```python
from build123d import *

# Parameters (mm, degrees)
RESSALTO_EXTRUS_O1_DEPTH     = 58
ESBO_O3_R                    = 2.75
RESSALTO_EXTRUS_O2_DEPTH     = 9
FILETE1_R                    = 5
FURO_DE_DI_METRO_0_15_14_1_D = 14
FUROAVAN_ADO1_OUTLINE_R      = 4.75
FUROAVAN_ADO1_DEPTH          = 9


# Read off the part's stored shape, not the designer's step: FuroAvançado1
with BuildPart() as part:
    # Esboço2 → Ressalto-extrusão1 (new body)
    with BuildSketch(Plane.XY):
        Polygon((-58, 0), (0, 0), (58, 0), (58, 9), (0, 9), (-58, 9), align=None)
    extrude(amount=-RESSALTO_EXTRUS_O1_DEPTH)

    # Esboço3 → Ressalto-extrusão2 (add)
    with BuildSketch(Plane(origin=(0, 9, 0), x_dir=(1, 0, 0), z_dir=(0, 1, 0))):
        with BuildLine():
            Line((-43.5, 42), (-24.799193535, 42))
            ThreePointArc((-24.799193535, 42), (0, 57), (24.799193535, 42))
            Line((24.799193535, 42), (43.5, 42))
            ThreePointArc((43.5, 42), (56.5, 29), (43.5, 16))
            Line((43.5, 16), (24.799193535, 16))
            ThreePointArc((24.799193535, 16), (0, 1), (-24.799193535, 16))
            Line((-24.799193535, 16), (-43.5, 16))
            ThreePointArc((-43.5, 16), (-56.5, 29), (-43.5, 42))
        make_face()
        with Locations(Location((-11, 42, 0), (0, 0, 270))):
            Circle(ESBO_O3_R, mode=Mode.SUBTRACT)
        with Locations(Location((11, 42, 0), (0, 0, 270))):
            Circle(ESBO_O3_R, mode=Mode.SUBTRACT)
        with Locations(Location((-11, 16, 0), (0, 0, 270))):
            Circle(ESBO_O3_R, mode=Mode.SUBTRACT)
        with Locations(Location((11, 16, 0), (0, 0, 270))):
            Circle(ESBO_O3_R, mode=Mode.SUBTRACT)
    extrude(amount=RESSALTO_EXTRUS_O2_DEPTH)

    # Filete1
    filete1_edges = [part.edges().sort_by_distance(p)[0] for p in [
        (24.799193535, 13.5, -42),
        (-24.799193535, 13.5, -42),
        (-24.799193535, 13.5, -16),
        (24.799193535, 13.5, -16),
    ]]
    fillet(filete1_edges, radius=FILETE1_R)

    # Furo de diâmetro Ø0.15 (14)1 (through all)
    with Locations(Plane(origin=(0, 18, 0), x_dir=(1, 0, 0), z_dir=(0, 1, 0))):
        with Locations((-43.5, 29), (43.5, 29)):
            Hole(FURO_DE_DI_METRO_0_15_14_1_D / 2)

    # FuroAvançado1 outline → FuroAvançado1 (cut)
    with BuildSketch(Plane(origin=(0, 0, 0), x_dir=(1, 0, 0), z_dir=(0, 1, 0))):
        with Locations((-11, 42)):
            Circle(FUROAVAN_ADO1_OUTLINE_R)
        with Locations((-11, 16)):
            Circle(FUROAVAN_ADO1_OUTLINE_R)
        with Locations((11, 16)):
            Circle(FUROAVAN_ADO1_OUTLINE_R)
        with Locations((11, 42)):
            Circle(FUROAVAN_ADO1_OUTLINE_R)
    extrude(amount=FUROAVAN_ADO1_DEPTH, mode=Mode.SUBTRACT)


solid = part.part
```
Model file for the job. Use its own axes, mm. A direction names the side the tool comes from. Coordinates: 2 decimals unless noted, no trailing zeros. Order: outer loops, then holes, each group sorted by start corner. A loop starts at its lowest first (then second) coordinate and runs counter-clockwise, first axis right, second up. Notation, with made-up numbers: (22, -37.75) - (81, -37.75) arc R19 cw to (81, -4.75) - close; hole circle Ø2 at (20, 79.25). An arc over 180 degrees is marked (long way). Return JSON: item names as keys, results as strings. Group by question number.
1) Probe line 1 (Z direction, x = -11, y = 7); line 2 (X direction, y = 6.25, z = -16); line 3 (X direction, y = 10.5, z = -18.5). List the from-to ranges inside material, lowest first. Write a range as from..to.
2) Saw through at A-A, the plane y = 15.5. Write the cut outline in (x, z).
3) Tool access for faces 1 (the flat face through (-8, 9, -16)), 2 (the flat face through (35, 13, -42)), 3 (the flat face through (-36, 13, -42)): list every direction of +Z, -Z, +X, -X, +Y, -Y with a clear straight run to the whole face (end or side of a thin tool).
4) Saw through at D-D, the plane z = -10. Write the cut outline in (x, y), plus the area to 3 significant figures.
5) Saw through at C-C, the plane z = -24.5. Write the cut outline in (x, y), plus the area to 3 significant figures.
6) Flat gauge pins, fed straight in: P1, Ø3, axis at x = -4.5, y = 11.5, coming from the +Z side; P2, Ø5, axis at x = 12, z = -17, coming from the -Y side; P3, Ø4.5, axis at x = -11, z = -42, coming from the +Y side; P4, Ø2.5, axis at x = -37, y = 14, coming from the -Z side. Where does each tip first touch, or does it go through?
7) Saw through at B-B, the plane x = 11. Write the cut outline in (y, z).
8) Mould opens along Z. For faces 4 (the cylindrical face through (10.38, 4.44, -20.71)), 5 (the cylindrical face through (25.244, 13.563, -15.379)), 6 (the cylindrical face through (-56.497, 13.437, -28.714)) say: released by +Z, released by -Z, zero draft, split by the parting line, or undercut.
Values found:
{
 "1": {"line 1": "z = -58..-46.75, -37.25..-20.75, -11.25..0", "line 2": "x = -58..-15.75, -6.25..6.25, 15.75..58", "line 3": "x = -51.16..-12.15, -9.85..9.85, 12.15..51.16"},
 "2": {"outline": "(-43.5, -42) - (-27.66, -42) arc R5 cw to (-23.47, -44.27) arc R28 ccw to (23.47, -44.27) arc R5 cw to (27.66, -42) - (43.5, -42) arc R13 ccw to (43.5, -16) - (27.66, -16) arc R5 cw to (23.47, -13.73) arc R28 ccw to (-23.47, -13.73) arc R5 cw to (-27.66, -16) - (-43.5, -16) arc R13 ccw to start; hole circle Ø14 at (-43.5, -29); hole circle Ø5.5 at (-11, -42); hole circle Ø5.5 at (-11, -16); hole circle Ø5.5 at (11, -42); hole circle Ø5.5 at (11, -16); hole circle Ø14 at (43.5, -29)"},
 "3": {"face 1": "-Y", "face 2": "-Z, +X, +Y", "face 3": "-Z, -X, +Y"},
 "4": {"outline": "(-58, 0) - (58, 0) - (58, 9) - (20.57, 9) - (20.57, 18) - (-20.57, 18) - (-20.57, 9) - (-58, 9) - close", "area": "1,410 mm²"},
 "5": {"outline": "(-58, 0) - (-48.86, 0) - (-48.86, 18) - (-55.7, 18) - (-55.7, 9) - (-58, 9) - close; (-38.14, 0) - (38.14, 0) - (38.14, 18) - (-38.14, 18) - close; (48.86, 0) - (58, 0) - (58, 9) - (55.7, 9) - (55.7, 18) - (48.86, 18) - close", "area": "1,660 mm²"},
 "6": {"P1": "stops at z = -1.16", "P2": "stops at y = 9", "P3": "passes through", "P4": "stops at z = -42"},
 "7": {"outline": "(0, -58) - (9, -58) - (9, -54.75) - (18, -54.75) - (18, -44.75) - (9, -44.75) - (9, -46.75) - (0, -46.75) - close; (0, -37.25) - (9, -37.25) - (9, -39.25) - (18, -39.25) - (18, -18.75) - (9, -18.75) - (9, -20.75) - (0, -20.75) - close; (0, -11.25) - (9, -11.25) - (9, -13.25) - (18, -13.25) - (18, -3.25) - (9, -3.25) - (9, 0) - (0, 0) - close"},
 "8": {"face 4": "undercut", "face 5": "released by +Z", "face 6": "split by the parting line"}
}
